Geometry: final body of the model. Coordinates: model frame, mm. Face numbers are marked on the shaded views. A direction names the side the tool comes from. Round coordinates to 2 decimals unless told otherwise and drop trailing zeros. Write each loop counter-clockwise with the first axis right and the second up, starting at its lowest first coordinate (ties: lowest second). Pieces come first, ordered by that corner, then holes. Notation, with made-up numbers: M -0.5,47.25 L 11.5,47.25 A27 cw 11.5,73.25 Z; hole C 26,6.25 d11. An arc over 180 degrees is marked long. Answer as CSV lines item,"result". Start each with the question number.
Q1. Reachability of the marked faces 1 and 2 from +Z, -Z, +X, -X, +Y, -Y: full face, straight path, thin tool, end or side. Return the list, or none.
Q2. Section query A-A on x = 0. Give the number of separate pieces and of enclosed holes in the cut face, and give its area (3 significant figures).
Q3. First-contact query: pin 1 (2 mm diameter, centred on x = -12.5, z = 1.5, fed in from -Y); pin 2 (1 mm diameter, centred on y = 48.5, z = 1.5, fed in from +X); pin 3 (8 mm diameter, centred on x = -11.5, y = 26, fed in from +Z). Flat tips, straight axial feed; report the tip coordinate or a pass-through.
Q4. Section query C-C on y = 26.25. Output: boundary loops of the cut face in (x, z), and give its area (3 significant figures).
Q5. Mould query, pull axis X, two halves, no side actions, for the marked faces 3, 4 and 5. Classes: pulls with the +X half, pulls with the -X half, needs draft (parallel to the pull), parting line crosses it, or undercut.
Q6. Ray query, probe 1 along Y at (x, z) = (0, 2.3); probe 2 along Y at (x, z) = (-11.5, 0.55); probe 3 along Z at (x, y) = (-14.5, 37). Return the intervals inside material, ascending.
Q7. Section query B-B on y = 33. Output: boundary loops of the cut face in (x, z).
```python
from build123d import *

# Parameters (mm, degrees)
EXTRUDE_1_DEPTH              = 3.6
CUT_EXTRUDE_1_DEPTH          = 2.1
CUT_EXTRUDE_2_DEPTH          = 2.1
CUT_EXTRUDE_3_DEPTH          = 2.1
CUT_EXTRUDE_4_DEPTH          = 2.1
CUT_EXTRUDE_5_DEPTH          = 2.1
SKETCH_7_W                   = 3.75
SKETCH_7_H                   = 2
HOLE_WIZARD_M3_1_D           = 3.3
HOLE_WIZARD_M3_1_CBORE_D     = 6
HOLE_WIZARD_M3_1_CBORE_DEPTH = 0.8
HOLE_WIZARD_3_4_3_4_1_D      = 3.4
HOLE_WIZARD_3_4_3_4_1_DEPTH  = 3.6
HOLE_WIZARD_M3_2_D           = 3.4
HOLE_WIZARD_M3_2_DEPTH       = 5.6
HOLE_WIZARD_M3_2_CBORE_D     = 6.5
HOLE_WIZARD_M3_2_CBORE_DEPTH = 2.1
HOLE_WIZARD_15_0_15_1_D      = 15
FILLET_1_R                   = 2


with BuildPart() as part:
    # 草图1 → 凸台-拉伸1 (new body)
    with BuildSketch(Plane(origin=(0, 0, 0), x_dir=(-1, 0, 0), z_dir=(0, 0, -1))):
        with BuildLine():
            Line((5, 0), (5, 16.229490169))
            ThreePointArc((5, 16.229490169), (0, 50.5), (-5, 16.229490169))
            Line((-5, 16.229490169), (-5, 0))
            ThreePointArc((-5, 0), (0, -5), (5, 0))
        make_face()
    extrude(amount=-EXTRUDE_1_DEPTH)

    # 草图2 → 切除-拉伸1 (cut)
    with BuildSketch(Plane(origin=(0, 0, 0), x_dir=(-1, 0, 0), z_dir=(0, 0, -1))):
        with BuildLine():
            Line((15.432267108, 27.842953181), (13.316342951, 29.064582562))
            ThreePointArc((13.316342951, 29.064582562), (8.876760389, 27.875), (10.066342951, 23.435417438))
            Line((10.066342951, 23.435417438), (12.182267108, 22.213788056))
            ThreePointArc((12.182267108, 22.213788056), (12.673627776, 21.478926775), (12.390283297, 20.641566449))
            ThreePointArc((12.390283297, 20.641566449), (15.155444566, 24.25), (16.897859054, 28.44891668))
            ThreePointArc((16.897859054, 28.44891668), (16.31435598, 27.784853001), (15.432267108, 27.842953181))
        make_face()
    extrude(amount=-CUT_EXTRUDE_1_DEPTH, mode=Mode.SUBTRACT)

    # 草图3 → 切除-拉伸2 (cut)
    with BuildSketch(Plane(origin=(0, 0, 0), x_dir=(-1, 0, 0), z_dir=(0, 0, -1))):
        with BuildLine():
            Line((12.182267108, 43.786211944), (10.066342951, 42.564582562))
            ThreePointArc((10.066342951, 42.564582562), (8.876760389, 38.125), (13.316342951, 36.935417438))
            Line((13.316342951, 36.935417438), (15.432267108, 38.157046819))
            ThreePointArc((15.432267108, 38.157046819), (16.31435598, 38.215146999), (16.897859054, 37.55108332))
            ThreePointArc((16.897859054, 37.55108332), (15.155444566, 41.75), (12.390283297, 45.358433551))
            ThreePointArc((12.390283297, 45.358433551), (12.673627776, 44.521073225), (12.182267108, 43.786211944))
        make_face()
    extrude(amount=-CUT_EXTRUDE_2_DEPTH, mode=Mode.SUBTRACT)

    # 草图4 → 切除-拉伸3 (cut)
    with BuildSketch(Plane(origin=(0, 0, 0), x_dir=(-1, 0, 0), z_dir=(0, 0, -1))):
        with BuildLine():
            Line((-3.25, 48.943258764), (-3.25, 46.5))
            ThreePointArc((-3.25, 46.5), (0, 43.25), (3.25, 46.5))
            Line((3.25, 46.5), (3.25, 48.943258764))
            ThreePointArc((3.25, 48.943258764), (3.640728204, 49.736220225), (4.507575758, 49.90951687))
            ThreePointArc((4.507575758, 49.90951687), (0, 50.5), (-4.507575758, 49.90951687))
            ThreePointArc((-4.507575758, 49.90951687), (-3.640728204, 49.736220225), (-3.25, 48.943258764))
        make_face()
    extrude(amount=-CUT_EXTRUDE_3_DEPTH, mode=Mode.SUBTRACT)

    # 草图5 → 切除-拉伸4 (cut)
    with BuildSketch(Plane(origin=(0, 0, 0), x_dir=(-1, 0, 0), z_dir=(0, 0, -1))):
        with BuildLine():
            Line((-15.432267108, 38.157046819), (-13.316342951, 36.935417438))
            ThreePointArc((-13.316342951, 36.935417438), (-8.876760389, 38.125), (-10.066342951, 42.564582562))
            Line((-10.066342951, 42.564582562), (-12.182267108, 43.786211944))
            ThreePointArc((-12.182267108, 43.786211944), (-12.673627776, 44.521073225), (-12.390283297, 45.358433551))
            ThreePointArc((-12.390283297, 45.358433551), (-15.155444566, 41.75), (-16.897859054, 37.55108332))
            ThreePointArc((-16.897859054, 37.55108332), (-16.31435598, 38.215146999), (-15.432267108, 38.157046819))
        make_face()
    extrude(amount=-CUT_EXTRUDE_4_DEPTH, mode=Mode.SUBTRACT)

    # 草图6 → 切除-拉伸5 (cut)
    with BuildSketch(Plane(origin=(0, 0, 0), x_dir=(-1, 0, 0), z_dir=(0, 0, -1))):
        with BuildLine():
            Line((-12.182267108, 22.213788056), (-10.066342951, 23.435417438))
            ThreePointArc((-10.066342951, 23.435417438), (-8.876760389, 27.875), (-13.316342951, 29.064582562))
            Line((-13.316342951, 29.064582562), (-15.432267108, 27.842953181))
            ThreePointArc((-15.432267108, 27.842953181), (-16.31435598, 27.784853001), (-16.897859054, 28.44891668))
            ThreePointArc((-16.897859054, 28.44891668), (-15.155444566, 24.25), (-12.390283297, 20.641566449))
            ThreePointArc((-12.390283297, 20.641566449), (-12.673627776, 21.478926775), (-12.182267108, 22.213788056))
        make_face()
    extrude(amount=-CUT_EXTRUDE_5_DEPTH, mode=Mode.SUBTRACT)

    # 草图7 → 旋转1 (revolve)
    with BuildSketch(Plane.XZ, mode=Mode.PRIVATE) as revolve_1_sk:
        with Locations((1.875, 4.6)):
            Rectangle(SKETCH_7_W, SKETCH_7_H)
    revolve(revolve_1_sk.sketch.rotate(Axis((0, 0, 5.6), (0, 0, -1)), 180), axis=Axis((0, 0, 5.6), (0, 0, -1)))

    # M3 六角头机械螺钉的柱形沉头孔1 (through all)
    with Locations(Plane(origin=(0, 0, 0), x_dir=(-1, 0, 0), z_dir=(0, 0, -1))):
        with Locations((0, 0)):
            CounterBoreHole(HOLE_WIZARD_M3_1_D / 2, HOLE_WIZARD_M3_1_CBORE_D / 2, HOLE_WIZARD_M3_1_CBORE_DEPTH)

    # Ø3.4 (3.4) 直径孔1
    with Locations(Plane.XY.offset(3.6)):
        with Locations((-11.691342951, 26.25), (-11.691342951, 39.75), (0, 46.5), (11.691342951, 39.75), (11.691342951, 26.25)):
            Hole(HOLE_WIZARD_3_4_3_4_1_D / 2, depth=HOLE_WIZARD_3_4_3_4_1_DEPTH)

    # M3 六角头机械螺钉的柱形沉头孔2
    with Locations(Plane(origin=(0, 0, 0), x_dir=(-1, 0, 0), z_dir=(0, 0, -1))):
        with Locations((0, 19.5)):
            CounterBoreHole(HOLE_WIZARD_M3_2_D / 2, HOLE_WIZARD_M3_2_CBORE_D / 2, HOLE_WIZARD_M3_2_CBORE_DEPTH, depth=HOLE_WIZARD_M3_2_DEPTH)

    # Ø15.0 (15) 直径孔1 (through all)
    with Locations(Plane.XY.offset(3.6)):
        with Locations((0, 33)):
            Hole(HOLE_WIZARD_15_0_15_1_D / 2)

    # 圆角1
    fillet_1_edges = [part.edges().sort_by_distance(p)[0] for p in [
        (5, 16.229490169, 1.8),
        (-5, 16.229490169, 1.8),
    ]]
    fillet(fillet_1_edges, radius=FILLET_1_R)


solid = part.part
```
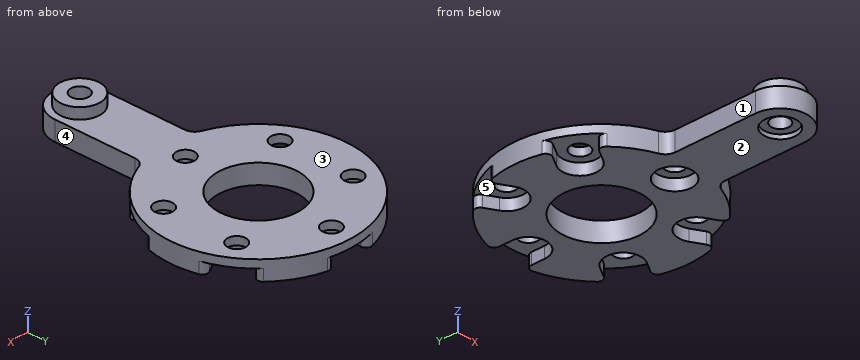
Entries:
1,face 1,"+Z, -Z, -X, -Y"
1,face 2,"-Z, +X, -X, +Y, -Y"
2,separate pieces,"5"
2,enclosed holes,"0"
2,area,"101 mm^2"
3,pin 1,"stops at y = 19.81"
3,pin 2,"stops at x = 9.01"
3,pin 3,"stops at z = 3.6"
4,outline,"M -16.15,2.1 L -13.39,2.1 L -13.39,3.6 L -16.15,3.6 Z; M -9.99,2.1 L -8.44,2.1 L -8.44,0 L -3.27,0 L -3.27,3.6 L -9.99,3.6 Z; M 3.27,0 L 8.44,0 L 8.44,2.1 L 9.99,2.1 L 9.99,3.6 L 3.27,3.6 Z; M 13.39,2.1 L 16.15,2.1 L 16.15,3.6 L 13.39,3.6 Z"
4,area,"50.2 mm^2"
5,face 3,"needs draft"
5,face 4,"pulls with the +X half"
5,face 5,"undercut"
6,probe 1,"y = -5 to -1.65, 1.65 to 17.8, 21.2 to 25.5, 40.5 to 44.8, 48.2 to 50.5"
6,probe 2,"y = 19.81 to 22.61, 29.49 to 36.51, 43.39 to 46.19"
6,probe 3,"z = 0 to 3.6"
7,outline,"M -17.5,0 L -7.5,0 L -7.5,3.6 L -17.5,3.6 Z; M 7.5,0 L 17.5,0 L 17.5,3.6 L 7.5,3.6 Z"
